Here's how the part is built. I have some questions about the finished solid (model axes, mm). Coordinates: 2 decimals unless noted, no trailing zeros. Loops run counter-clockwise (first coordinate to the right, second up) from the corner with the lowest first, then second, coordinate; pieces in that order, holes last.
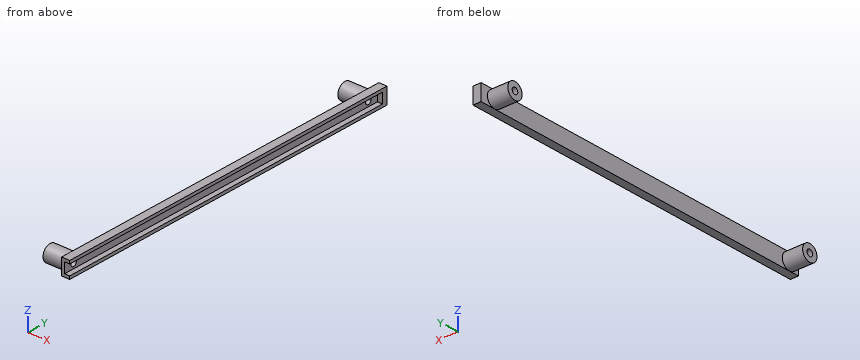
Autodesk Inventor part; units mm, degrees
ref_plane "YZ Plane" through (0, 0, 0) normal (1, 0, 0) x (0, 1, 0)
ref_plane "XZ Plane" through (0, 0, 0) normal (0, 1, 0) x (-1, 0, 0)
ref_plane "XY Plane" through (0, 0, 0) normal (0, 0, 1) x (1, 0, 0)
sketch "Sketch1" plane through (0, 0, 0) normal (0, 1, 0) x (-1, 0, 0)
  line L0 (0, 3.1877) -> (3.1877, 3.1877)
  line L1 (3.1877, 3.1877) -> (3.1877, -3.175)
  line L2 (3.1877, -3.175) -> (0, -3.175)
  line L3 (0, 5.08) -> (5.08, 5.08)
  line L4 (5.08, 5.08) -> (5.08, -5.08)
  line L5 (5.08, -5.08) -> (0, -5.08)
  line L6 (0, -5.08) -> (0, -3.175)
  line L7 (0, 3.1877) -> (0, 5.08)
  point P0 (0, 0)
  dimension "d0" = 3.1877
  dimension "d1" = 5.08
  dimension "d2" = 10.16
extrude "Extrusion1" add sketch "Sketch1" along normal blind 221.4118
sketch "Sketch2" plane through (-5.08, 0, -5.08) normal (-1, 0, 0) x (0, 0, 1)
  circle A0 centre (5.08, 6.35) radius 1.9844
  circle A1 centre (5.08, 215.0618) radius 1.9844
  point P0 (5.08, 0)
  dimension "d5" = 3.9688
  dimension "d6" = 3.9688
extrude "Extrusion2" cut sketch "Sketch2" against normal blind 221.4118
sketch "Sketch3" plane through (-5.08, 0, -5.08) normal (-1, 0, 0) x (0, 0, 1)
  circle A0 centre (5.08, 6.35) radius 5.08
  circle A1 centre (5.08, 215.0618) radius 1.9844
  circle A2 centre (5.08, 215.0618) radius 5.08
  line L0 (10.16, 0) -> (10.16, 221.4118)
  circle A3 centre (5.08, 6.35) radius 1.9844
  point P0 (5.08, 0)
  dimension "d9" = 10.16
extrude "Extrusion3" add sketch "Sketch3" along normal blind 12.7
sketch "Sketch4" plane through (0, 221.4118, 0) normal (0, 1, 0) x (1, 0, 0)
  line L0 (-5.08, -5.08) -> (0, -5.08)
  line L1 (-5.08, -5.08) -> (-5.08, 5.08)
  line L2 (0, -5.08) -> (-5.08, -5.08)
  line L3 (-5.08, -5.08) -> (-5.08, 5.08)
  line L4 (-5.08, 5.08) -> (0, 5.08)
  line L5 (0, 5.08) -> (0, -5.08)
  point P0 (0, 0)
extrude "Extrusion4" add sketch "Sketch4" along normal blind 3.175
sketch "Sketch5" plane through (-5.08, 6.35, -5.08) normal (-1, 0, 0) x (0, 0, 1)
  point P0 (5.08, -6.35)
properties part number "hs_intake_synchronizer"
1. I want a section at B-B (z = 0). Please give me the cut outline in (x, y), then the cut area to 3 significant figures.
2. I want a section at A-A (x = -14.5). Please give me the cut outline in (y, z), then the cut area to 3 significant figures.
3. For pin 1 (4 mm diameter, centred on x = -11.5, z = 2, fed in from +Y); pin 2 (1.5 mm diameter, centred on y = 74, z = -1.5, fed in from +X); pin 3 (3 mm diameter, centred on y = 147, z = -1, fed in from -X), each with a flat end and sliding along its axis, tell me the tip position at first contact or that it passes through.
4. I need wall thicknesses on line 1 along Y through (x, z) = (-11.25, 0); line 2 along Z through (x, y) = (-1.5, 183) (3 decimals); line 3 along Y through (x, z) = (-14, 1.5). Which ranges of each line are inside material? Lowest first, please.
5. I want a section at C-C (y = 192.5). Please give me the cut outline in (x, z) (3 decimals), then the cut area to 3 significant figures.
Response values:
1. outline: (-17.78, 1.27) - (-5.08, 1.27) - (-5.08, 0) - (-3.19, 0) - (-3.19, 4.37) - (-17.78, 4.37) - close; (-17.78, 8.33) - (-3.19, 8.33) - (-3.19, 213.08) - (-17.78, 213.08) - (-17.78, 209.98) - (-5.08, 209.98) - (-5.08, 11.43) - (-17.78, 11.43) - close; (-17.78, 217.05) - (-3.19, 217.05) - (-3.19, 221.41) - (0, 221.41) - (0, 224.59) - (-5.08, 224.59) - (-5.08, 220.14) - (-17.78, 220.14) - close
1. area: 577 mm2
2. outline: circle Ø10.16 at (6.35, 0); circle Ø10.16 at (215.06, 0); hole circle Ø3.97 at (6.35, 0); hole circle Ø3.97 at (215.06, 0)
2. area: 137 mm2
3. pin 1: stops at y = 220.14
3. pin 2: stops at x = -3.19
3. pin 3: stops at x = -5.08
4. line 1: y = 1.27 to 4.37, 8.33 to 11.43, 209.98 to 213.08, 217.05 to 220.14
4. line 2: z = -5.08 to -3.175, 3.188 to 5.08
4. line 3: y = 1.5 to 5.05, 7.65 to 11.2, 210.21 to 213.76, 216.36 to 219.92
5. outline: (-5.08, -5.08) - (0, -5.08) - (0, -3.175) - (-3.188, -3.175) - (-3.188, 3.188) - (0, 3.188) - (0, 5.08) - (-5.08, 5.08) - close
5. area: 31.3 mm2
